Autodesk Inventor part; units mm, degrees
ref_plane "YZ Plane" through (0, 0, 0) normal (1, 0, 0) x (0, 1, 0)
ref_plane "XZ Plane" through (0, 0, 0) normal (0, 1, 0) x (-1, 0, 0)
ref_plane "XY Plane" through (0, 0, 0) normal (0, 0, 1) x (1, 0, 0)
sketch "Sketch1" plane through (0, 0, 0) normal (1, 0, 0) x (0, 1, 0)
  circle A0 centre (0, 0) radius 16
  circle A1 centre (0, 0) radius 13.5
  dimension "d0" = 32
  dimension "d1" = 27
extrude "Extrusion1" add sketch "Sketch1" along normal mid plane 355
sketch "Sketch2" plane through (177.5, 0, 0) normal (1, 0, 0) x (0, 0, -1)
  circle A0 centre (0, 0) radius 16
  dimension "d4" = 32
extrude "Extrusion2" add sketch "Sketch2" along normal blind 5
sketch "Sketch3" plane through (-177.5, 0, 0) normal (-1, 0, 0) x (0, 0, 1)
  circle A0 centre (0, 0) radius 16
extrude "Extrusion3" add sketch "Sketch3" along normal blind 5
properties material "Glass"
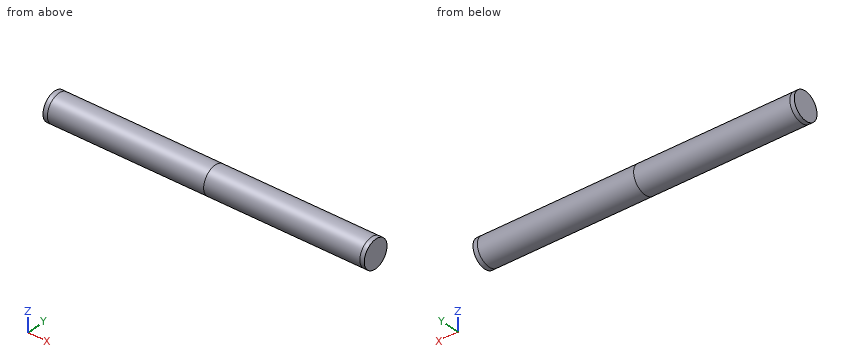
The model under review builds one solid part; all positions refer to its coordinate system, in mm. Round coordinates to 2 decimals unless told otherwise and drop trailing zeros. Loops run counter-clockwise (first coordinate to the right, second up) from the corner with the lowest first, then second, coordinate; pieces in that order, holes last.
1) Wall thickness on line 1 along Z through (x, y) = (-41.5, 0); line 2 along X through (y, z) = (-8.5, 0.5); line 3 along Z through (x, y) = (-76, 1.5): over which ranges is each line inside the solid? List them lowest first.
Values follow:
line 1: z = -16 to -13.5, 13.5 to 16
line 2: x = -182.5 to -177.5, 177.5 to 182.5
line 3: z = -15.93 to -13.42, 13.42 to 15.93
2) Consider section C-C on x = 80.5. State the section outline as (y, z) points, then the cut area to 3 significant figures.
Values follow:
outline: circle Ø32 at (0, 0); hole circle Ø27 at (0, 0)
area: 232 mm2
3) Consider section A-A on y = 0. State the section outline as (x, z) points.
Values follow:
outline: (-182.5, -16) - (182.5, -16) - (182.5, 16) - (-182.5, 16) - close; hole (-177.5, -13.5) - (177.5, -13.5) - (177.5, 13.5) - (-177.5, 13.5) - close
4) Clearance check with flat-ended pins moving along their axes: P1, Ø1.5, axis at x = 135, y = -4.5, coming from the -Z side; P2, Ø6, axis at x = 73, y = 4.5, coming from the -Z side; P3, Ø3, axis at x = -113.5, z = -5.5, coming from the -Y side. State where each tip first meets the part, or that it passes through.
Values follow:
P1: stops at z = -15.55
P2: stops at z = -15.93
P3: stops at y = -15.49
